Here's how the part is built. I have some questions about the finished solid (model axes, mm). Coordinates: 2 decimals unless noted, no trailing zeros. Write each loop counter-clockwise with the first axis right and the second up, starting at its lowest first coordinate (ties: lowest second). Pieces come first, ordered by that corner, then holes.
Item 1: I want a section at C-C (z = -36). Please give me the cut outline in (x, y).
Item 2: I'm going to push flat-ended pins straight in: P1, Ø4, axis at x = 6, z = -25, coming from the +Y side; P2, Ø3, axis at y = 12.5, z = -39, coming from the -X side; P3, Ø5, axis at y = 17.5, z = -21.5, coming from the -X side. Where does each tip first touch, or does it pass through?
Item 3: If we mould it in two halves opening along X, with no side actions, what happens to faces 1 (the face through (-1.365, 10.393, 16.79)), 2 (the face through (6.904, -13.274, 16.79)), 3 (the face through (0, -13, -50.732))? For each: pulls with the +X half, pulls with the -X half, needs draft (parallel to the pull), parting line crosses it, or undercut.
Item 4: Please list where these lines run through material, in increasing order: line 1 (Y direction, x = 0, z = 17); line 2 (Y direction, x = -2.5, z = -23); line 3 (X direction, y = 2.5, z = -14).
Item 5: I want a section at D-D (z = -45). Please give me the cut outline in (x, y).
from build123d import *

# Parameters (mm, degrees)
F2_R     = 10.5
F3_DEPTH = 90.17
F4_R     = 14.962462
F4_R_2   = 10.482231
F5_DEPTH = 25.4


with BuildPart() as f1:
    # F0 (on Front) → F1 (revolve)
    with BuildSketch(Plane.XZ):
        Polygon((0, -50.732268), (0, 4.267732), (-15, 4.267732), (-30, -50.732268), align=None)
    revolve(axis=Axis((0, 0, -23.232268), (0, 0, -1)))

    # F2 (on face) → F3 (cut)
    with BuildSketch(Plane.XY.offset(4.267732)):
        Circle(F2_R)
    extrude(amount=-F3_DEPTH, mode=Mode.SUBTRACT)

    # F4 (on face) → F5 (join)
    with BuildSketch(Plane.XY.offset(4.267732)):
        Circle(F4_R)
        Circle(F4_R_2, mode=Mode.SUBTRACT)
    extrude(amount=F5_DEPTH)


solid = f1.part
Answer:
1. outline: circle Ø51.96 at (0, 0); hole circle Ø21 at (0, 0)
2. P1: stops at y = 22.92
2. P2: stops at x = -24.57
2. P3: stops at x = -16.31
3. face 1: undercut
3. face 2: parting line crosses it
3. face 3: needs draft
4. line 1: y = -14.96 to -10.48, 10.48 to 14.96
4. line 2: y = -22.3 to -10.2, 10.2 to 22.3
4. line 3: x = -19.83 to -10.2, 10.2 to 19.83
5. outline: circle Ø56.87 at (0, 0); hole circle Ø21 at (0, 0)
